Can you work these out from the model? Positions are in its coordinate system, mm. A direction names the side the tool comes from. Coordinates: 2 decimals unless noted, no trailing zeros. Loops run counter-clockwise (first coordinate to the right, second up) from the corner with the lowest first, then second, coordinate; pieces in that order, holes last. Notation, with made-up numbers: M 30.5,-2 L 76.5,-2 A15 cw 76.5,16 Z; hole C 37.25,-22.75 d8. An arc over 180 degrees is marked long. Answer as a JSON object with one key per item and string values. Group by question number.
Item 1: We'd pull the mould along Z, two halves only. Please class faces 3 (the cylindrical face through (2.262, -0.712, -2.389)), 4 (the flat face through (4.3, 4.3, 0.8)), 5 (the cylindrical face through (2.262, -0.712, -4.861)), 6 (the flat face through (0, 0, 2.032)): +Z half, -Z half, draft (parallel to the pull), parting line (faces both ways), or undercut.
Item 2: Suppose I cut it at C-C (z = 1.25). Write out the boundary of the cut face in (x, y), then the cut area to 3 significant figures.
Item 3: Which directions (+Z, -Z, +X, -X, +Y, -Y) give clear straight access to the entire face, cutting with the end or side of a thin tool? Please do faces 1 (the flat face through (0, 0, -6.7)), 2 (the cylindrical face through (-1.266, 5.703, 0.394)).
Item 4: Suppose I cut it at A-A (y = 0). Write out the boundary of the cut face in (x, z).
Item 5: I'm going to push flat-ended pins straight in: pin 1 Ø1.5 at (y, z) = (-1.5, -3) entering from +X; pin 2 Ø1.5 at (x, y) = (-7, 3) entering from -Z; pin 3 Ø3 at (x, z) = (4.5, -3.5) entering from -Y. Where does each tip first touch, or does it pass through?
Item 6: If I drill on line 1 (Z direction, x = -4.25, y = 1.5); line 2 (Z direction, x = -5.5, y = -3); line 3 (Y direction, x = 0, z = -1.75), over which ranges is the centre line in solid material (lowest first)?
```python
from build123d import *

# Parameters (mm, degrees)
F2_SIZE  = 1.27
F3_R     = 14.2800405429
F3_R_2   = 10
F3_R_3   = 5.842
F4_DEPTH = 0.8
F5_SIZE  = 1.016


# Not quite as in the source:
# - a fillet or chamfer that OpenCascade refuses, or shapes differently, is made with other operations: its cross-section is extruded or revolved along the edge and cut away or added


with BuildPart() as f1:
    # F0 (on Front) → F1 (revolve)
    with BuildSketch(Plane.XZ):
        with BuildLine():
            Line((2.6757909362, 0), (4.2185683136, 0))
            Line((4.2185683136, 0), (10, 0))
            Line((10, 0), (10, 2.032))
            Line((10, 2.032), (0, 2.032))
            Line((0, 2.032), (0, 0))
            Line((0, 0), (0, -6.7))
            Line((0, -6.7), (2.3710267587, -6.7))
            Line((2.3710267587, -6.7), (2.3710267587, -4.308))
            ThreePointArc((2.3710267587, -4.308), (2.6250267587, -4.054), (2.3710267587, -3.8))
            Line((2.3710267587, -3.8), (2.3710267587, 0))
            Line((2.3710267587, 0), (2.6757909362, 0))
        make_face()
    revolve(axis=Axis((0, 0, 1.016), (0, 0, -1)))

    # F2
    f2_edges = [f1.edges().sort_by_distance(p)[0] for p in [
        (-2.371027, 0, -6.7),
    ]]
    chamfer(f2_edges, length=F2_SIZE)

    # F3 (on face) → F4 (cut)
    with BuildSketch(Plane(origin=(0, 0, 0), x_dir=(1, 0, 0), z_dir=(0, 0, -1))):
        Circle(F3_R)
        Circle(F3_R_2, mode=Mode.SUBTRACT)
        Circle(F3_R_2)
        Circle(F3_R_3, mode=Mode.SUBTRACT)
    extrude(amount=-F4_DEPTH, mode=Mode.SUBTRACT)

    # F5
    f5_edges = [f1.edges().sort_by_distance(p)[0] for p in [
        (-2.371027, 0, 0),
    ]]
    chamfer(f5_edges, length=F5_SIZE)

    # F6: chamfer of 1.27 on 1 edges, made by hand

    # F6_s1 → F6_t2 (revolve, cut)
    with BuildSketch(Plane.XZ):
        Polygon((10, 0.762), (8.73, 2.032), (10, 2.032), align=None)
    revolve(axis=Axis((0, 0, 2.032), (0, 0, -1)), mode=Mode.SUBTRACT)


solid = f1.part
```
From the geometry:
{
 "1": {"face 3": "undercut", "face 4": "-Z half", "face 5": "draft", "face 6": "+Z half"},
 "2": {"outline": "C 0,0 d19.02", "area": "284 mm2"},
 "3": {"face 1": "-Z, +X, -X, +Y, -Y", "face 2": "-Z"},
 "4": {"outline": "M -9.96,0.8 L -5.84,0.8 L -5.84,0 L -3.39,0 L -2.37,-1.02 L -2.37,-3.8 A0.25 ccw -2.37,-4.31 L -2.37,-5.43 L -1.1,-6.7 L 1.1,-6.7 L 2.37,-5.43 L 2.37,-4.31 A0.25 ccw 2.37,-3.8 L 2.37,-1.02 L 3.39,0 L 5.84,0 L 5.84,0.8 L 9.96,0.8 L 8.73,2.03 L -8.73,2.03 Z"},
 "5": {"pin 1": "x = 2.25", "pin 2": "z = 0.8", "pin 3": "through"},
 "6": {"line 1": "0 to 2.03", "line 2": "0.8 to 2.03", "line 3": "-2.37 to 2.37"}
}
